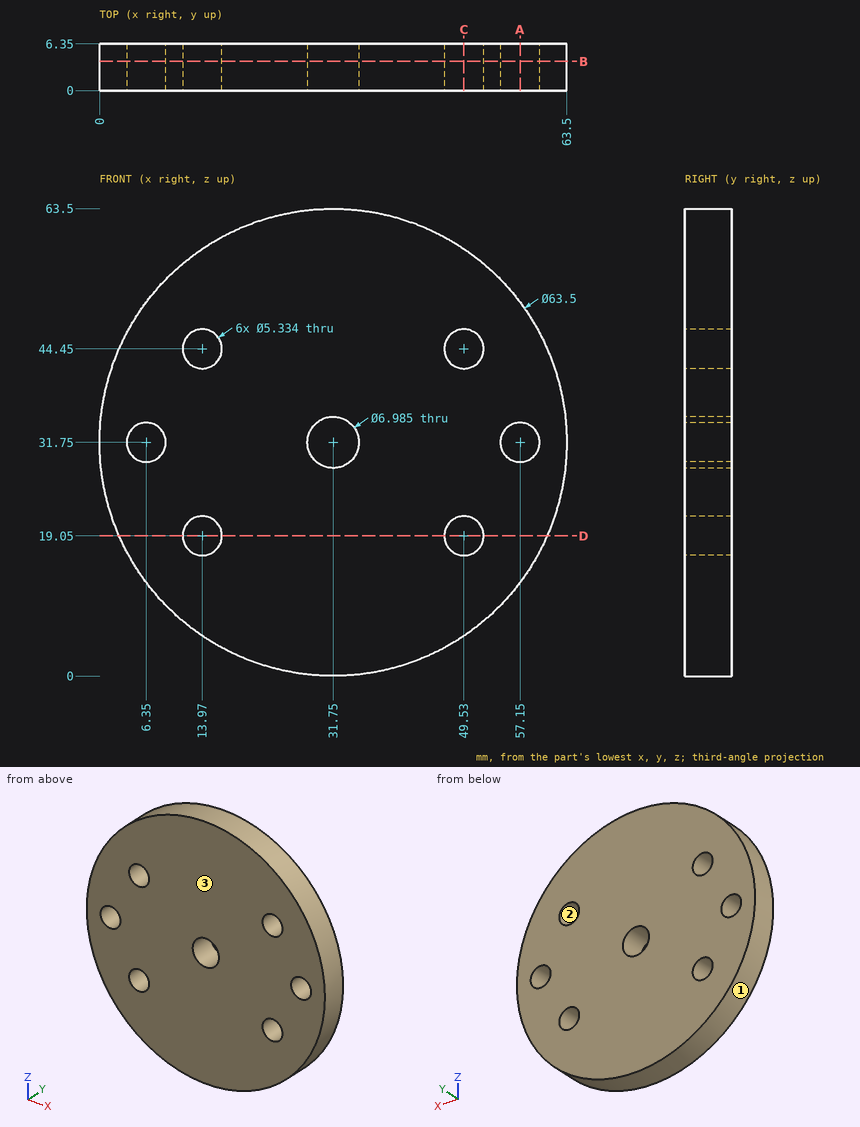
Input: dimensioned drawing with shaded views. Units: mm. Origin: part minimum x, y, z. Round coordinates to 2 decimals unless told otherwise and drop trailing zeros. Loops run counter-clockwise (first coordinate to the right, second up) from the corner with the lowest first, then second, coordinate; pieces in that order, holes last. Notation, with made-up numbers: M 31.25,84 L 60.25,84 A15 ccw 60.25,88 Z; hole C 67,-37.5 d4. An arc over 180 degrees is marked long. Return JSON: item names as keys, results as strings. Group by question number.
1. Section query D-D on z = 19.05. Output: boundary loops of the cut face in (x, y), and give its area (3 significant figures).
2. Material intervals for line 1 along Z through (x, y) = (49.5, 3.5); line 2 along Z through (x, y) = (6.35, 2.25); line 3 along X through (y, z) = (3.25, 15), sorted ascending. Write a range as from..to.
3. Pin query (flat end, axial travel): pin 1 (1.5 mm diameter, centred on y = 1, z = 20.5, fed in from -X); pin 2 (3 mm diameter, centred on x = 8.5, y = 0.5, fed in from -Z); pin 3 (5 mm diameter, centred on x = 49.53, z = 44.45, fed in from -Y). Return the tip coordinate at first contact, or that it passes through.
4. Section query C-C on x = 49.53. Output: boundary loops of the cut face in (y, z), and give its area (3 significant figures).
5. Mould query, pull axis X, two halves, no side actions, for the marked faces 1, 2 and 3. Classes: released by +X, released by -X, zero draft, split by the parting line, or undercut.
6. Section query B-B on y = 4. State how many separate pieces and enclosed holes the cut face has, and give its area (3 significant figures).
7. Section query A-A on x = 57.15. Output: boundary loops of the cut face in (y, z).
Checks:
{
 "1": {"outline": "M 2.65,0 L 11.3,0 L 11.3,6.35 L 2.65,6.35 Z; M 16.64,0 L 46.86,0 L 46.86,6.35 L 16.64,6.35 Z; M 52.2,0 L 60.85,0 L 60.85,6.35 L 52.2,6.35 Z", "area": "302 mm²"},
 "2": {"line 1": "z = 5.43..16.38, 21.72..41.78, 47.12..58.07", "line 2": "z = 12.7..29.08, 34.42..50.8", "line 3": "x = 4.78..58.72"},
 "3": {"pin 1": "stops at x = 1.79", "pin 2": "stops at z = 8.62", "pin 3": "passes through"},
 "4": {"outline": "M 0,5.45 L 6.35,5.45 L 6.35,16.38 L 0,16.38 Z; M 0,21.72 L 6.35,21.72 L 6.35,41.78 L 0,41.78 Z; M 0,47.12 L 6.35,47.12 L 6.35,58.05 L 0,58.05 Z", "area": "266 mm²"},
 "5": {"face 1": "split by the parting line", "face 2": "undercut", "face 3": "zero draft"},
 "6": {"separate pieces": "1", "enclosed holes": "7", "area": "2,990 mm²"},
 "7": {"outline": "M 0,12.7 L 6.35,12.7 L 6.35,29.08 L 0,29.08 Z; M 0,34.42 L 6.35,34.42 L 6.35,50.8 L 0,50.8 Z"}
}
